```python
from build123d import *

# Parameters (mm, degrees)
F0_W        = 6.35
F0_H        = 106.68
F1_DEPTH    = 1.5875
F2_T1_DEPTH = 20.6375
F3_T1_DEPTH = 20.6375


# Not quite as in the source:
# - a fillet or chamfer that OpenCascade refuses, or shapes differently, is made with other operations: its cross-section is extruded or revolved along the edge and cut away or added


with BuildPart() as f1:
    # F0 (on Front) → F1 (new body)
    with BuildSketch(Plane.XZ):
        with Locations((-32.9172081137, -12.1981453611)):
            Rectangle(F0_W, F0_H)
    extrude(amount=F1_DEPTH)

    # F2: fillet of radius 3.81 on 2 edges, made by hand

    # F2_s2 → F2_t1 (cut)
    with BuildSketch(Plane.XZ.offset(-9.525)):
        with BuildLine():
            ThreePointArc((-36.0922081137, 37.3318546389), (-34.97628495, 40.0259314752), (-32.2822081137, 41.1418546389))
            Line((-32.2822081137, 41.1418546389), (-36.0922081137, 41.1418546389))
            Line((-36.0922081137, 41.1418546389), (-36.0922081137, 37.3318546389))
        make_face()
        with BuildLine():
            ThreePointArc((-29.7422081137, 37.3318546389), (-30.8581312774, 40.0259314752), (-33.5522081137, 41.1418546389))
            Line((-33.5522081137, 41.1418546389), (-29.7422081137, 41.1418546389))
            Line((-29.7422081137, 41.1418546389), (-29.7422081137, 37.3318546389))
        make_face()
    extrude(amount=F2_T1_DEPTH, mode=Mode.SUBTRACT)

    # F3: fillet of radius 3.81 on 2 edges, made by hand

    # F3_s2 → F3_t1 (cut)
    with BuildSketch(Plane.XZ.offset(-9.525)):
        with BuildLine():
            ThreePointArc((-36.0922081137, -61.7281453611), (-34.97628495, -64.4222221974), (-32.2822081137, -65.5381453611))
            Line((-32.2822081137, -65.5381453611), (-36.0922081137, -65.5381453611))
            Line((-36.0922081137, -65.5381453611), (-36.0922081137, -61.7281453611))
        make_face()
        with BuildLine():
            ThreePointArc((-33.5522081137, -65.5381453611), (-30.8581312774, -64.4222221974), (-29.7422081137, -61.7281453611))
            Line((-29.7422081137, -61.7281453611), (-29.7422081137, -65.5381453611))
            Line((-29.7422081137, -65.5381453611), (-33.5522081137, -65.5381453611))
        make_face()
    extrude(amount=F3_T1_DEPTH, mode=Mode.SUBTRACT)


solid = f1.part
```
Here's how the part is built. I have some questions about the finished solid (model axes, mm). Coordinates: 2 decimals unless noted, no trailing zeros. Order: outer loops, then holes, each group sorted by start corner. A loop starts at its lowest first (then second) coordinate and runs counter-clockwise, first axis right, second up.
Item 1: If we section it at B-B, the plane x = -31: List the corners of the cut face in (y, z) for me, then the cut area to 3 significant figures.
Response values:
outline: (-1.59, -64.56) - (0, -64.56) - (0, 40.16) - (-1.59, 40.16) - close
area: 166 mm2
Item 2: If we section it at A-A, the plane y = -0.25: List the corners of the cut face in (x, z) for me, then the cut area to 3 significant figures.
Response values:
outline: (-36.09, -61.73) arc R3.81 ccw to (-32.92, -65.48) arc R3.81 ccw to (-29.74, -61.73) - (-29.74, 37.33) arc R3.81 ccw to (-32.92, 41.09) arc R3.81 ccw to (-36.09, 37.33) - close
area: 665 mm2
Item 3: I'm going to push a flat-ended pin straight in: pin 1 Ø3 at (x, z) = (-32.5, 4.5) entering from +Y. Where does the tip first touch, or does it pass through?
Response values:
pin 1: stops at y = 0
Item 4: I need wall thicknesses on probe 1 along Z at (x, y) = (-33, -0.1); probe 2 along Z at (x, y) = (-33.25, -0.3). Which ranges of each line are inside material? Lowest first, please.
Response values:
probe 1: z = -65.47 to 41.07
probe 2: z = -65.41 to 41.02
